Design review of the part built by this model. Coordinates are the model's own, in mm. Give positions to 0.01 mm unless a question says otherwise; leave off trailing zeros. Order: outer loops, then holes, each group sorted by start corner. A loop starts at its lowest first (then second) coordinate and runs counter-clockwise, first axis right, second up. Notation, with made-up numbers: M 1,29.25 L 35,29.25 A24 cw 35,43.25 Z; hole C 30.25,-27 d3. An arc over 180 degrees is marked long. Put each result on its own line as item: value. Start each with the question number.
from build123d import *

# Parameters (mm, degrees)
F1_DEPTH = 38.1


with BuildPart() as f1:
    # F0 (on Right) → F1 (new body)
    with BuildSketch(Plane.YZ):
        with BuildLine():
            Line((-444.5, 0), (0, 0))
            Line((0, 0), (0, 38.1))
            Line((0, 38.1), (-416.537181, 29.174203))
            ThreePointArc((-416.537181, 29.174203), (-436.345868, 20.593727), (-444.5, 0.605762))
            Line((-444.5, 0.605762), (-444.5, 0))
        make_face()
    extrude(amount=F1_DEPTH)


solid = f1.part
1. Consider section B-B on y = -70. Give the boundary of the cut face in (x, z).
2. Consider section A-A on x = 10. Give the boundary of the cut face in (y, z) (3 decimals), then the cut area to 3 significant figures.
3. To check wall thickness, follow probe 1 along Z at (x, y) = (33, -45); probe 2 along Y at (x, z) = (35.5, 4.5); probe 3 along Z at (x, y) = (23.5, -266). State the ranges of each line that lie inside material, in increasing order.
4. Insertion check: pin 1 (12 mm diameter, centred on x = 27.5, z = 15, fed in from -Y); pin 2 (12 mm diameter, centred on x = 30, y = -177, fed in from +Z); pin 3 (4 mm diameter, centred on x = 23.5, y = -150, fed in from +Z). Each pin has a flat end and moves straight along its axis. Give the tip position at first contact, or say it passes through.
5. Consider section C-C on z = 22. Give the boundary of the cut face in (x, y).
Returned:
1. outline: M 0,0 L 38.1,0 L 38.1,36.6 L 0,36.6 Z
2. outline: M -444.5,0 L 0,0 L 0,38.1 L -416.537,29.174 A28.575 ccw -444.5,0.606 Z
2. area: 14,700 mm2
3. probe 1: z = 0 to 37.14
3. probe 2: y = -444.23 to 0
3. probe 3: z = 0 to 32.4
4. pin 1: stops at y = -443.24
4. pin 2: stops at z = 34.44
4. pin 3: stops at z = 34.93
5. outline: M 0,-434.87 L 38.1,-434.87 L 38.1,0 L 0,0 Z
